from build123d import *

# Parameters (mm, degrees)
CROQUIS3_W                   = 38
CROQUIS3_H                   = 38
SALIENTE_EXTRUIR9_DEPTH      = 1
SALIENTE_EXTRUIR10_START     = -11
SALIENTE_EXTRUIR10_OUTLINE_W = 38
SALIENTE_EXTRUIR10_OUTLINE_H = 38
SALIENTE_EXTRUIR10_DEPTH     = 10
REDONDEO3_R                  = 1
CROQUIS13_W                  = 38
CROQUIS13_H                  = 38
SALIENTE_EXTRUIR15_DEPTH     = 3
CROQUIS15_R                  = 1.5
CORTAR_EXTRUIR5_DEPTH        = 5


# Read off the part's stored shape, not the designer's step: Saliente-Extruir10
with BuildPart() as part:
    # Croquis3 → Saliente-Extruir9 (new body)
    with BuildSketch(Plane.XY.offset(5)):
        Polygon((19, -5.370057685), (26.870057685, 2.5), (26.870057685, 40.5), (19, 48.370057685), (-19, 48.370057685), (-26.870057685, 40.5), (-26.870057685, 2.5), (-19, -5.370057685), align=None)
        with Locations((0, 21.5)):
            Rectangle(CROQUIS3_W, CROQUIS3_H, mode=Mode.SUBTRACT)
    extrude(amount=-SALIENTE_EXTRUIR9_DEPTH)

    # Saliente-Extruir10 outline → Saliente-Extruir10 (add)
    with BuildSketch(Plane(origin=(0, 0, 4), x_dir=(-1, 0, 0), z_dir=(0, 0, -1)).offset(SALIENTE_EXTRUIR10_START)):
        Polygon((-26.870057685, 2.5), (-19, -5.370057685), (19, -5.370057685), (26.870057685, 2.5), (26.870057685, 40.5), (19, 48.370057685), (-19, 48.370057685), (-26.870057685, 40.5), align=None)
        with Locations((0, 21.5)):
            Rectangle(SALIENTE_EXTRUIR10_OUTLINE_W, SALIENTE_EXTRUIR10_OUTLINE_H, mode=Mode.SUBTRACT)
    extrude(amount=SALIENTE_EXTRUIR10_DEPTH)

    # Redondeo3
    redondeo3_edges = [part.edges().sort_by_distance(p)[0] for p in [
        (-19, 48.370057685, 10),
        (19, 48.370057685, 10),
    ]]
    fillet(redondeo3_edges, radius=REDONDEO3_R)

    # Croquis13 → Saliente-Extruir15 (add)
    with BuildSketch(Plane.XY.offset(15)):
        with BuildLine():
            Line((-22.5, 44.870057685), (-22.5, -1))
            Line((-22.5, -1), (22.5, -1))
            Line((22.5, -1), (22.5, 44.870057685))
            Line((22.5, 44.870057685), (19.292893219, 48.077164466))
            ThreePointArc((19.292893219, 48.077164466), (18.96846987, 48.293937218), (18.585786438, 48.370057685))
            Line((18.585786438, 48.370057685), (-18.585786438, 48.370057685))
            ThreePointArc((-18.585786438, 48.370057685), (-18.96846987, 48.293937218), (-19.292893219, 48.077164466))
            Line((-19.292893219, 48.077164466), (-22.5, 44.870057685))
        make_face()
        with Locations((0, 21.5)):
            Rectangle(CROQUIS13_W, CROQUIS13_H, mode=Mode.SUBTRACT)
    extrude(amount=SALIENTE_EXTRUIR15_DEPTH)

    # Croquis15 → Cortar-Extruir5 (cut)
    with BuildSketch(Plane(origin=(0, 48.370057685, 0), x_dir=(1, 0, 0), z_dir=(0, 1, 0))):
        with Locations(Location((0, -12.5, 0), (0, 0, 270))):
            Circle(CROQUIS15_R)
        with Locations(Location((-10, -12.5, 0), (0, 0, 270))):
            Circle(CROQUIS15_R)
        with Locations(Location((10, -12.5, 0), (0, 0, 90))):
            Circle(CROQUIS15_R)
    extrude(amount=-CORTAR_EXTRUIR5_DEPTH, mode=Mode.SUBTRACT)


solid = part.part
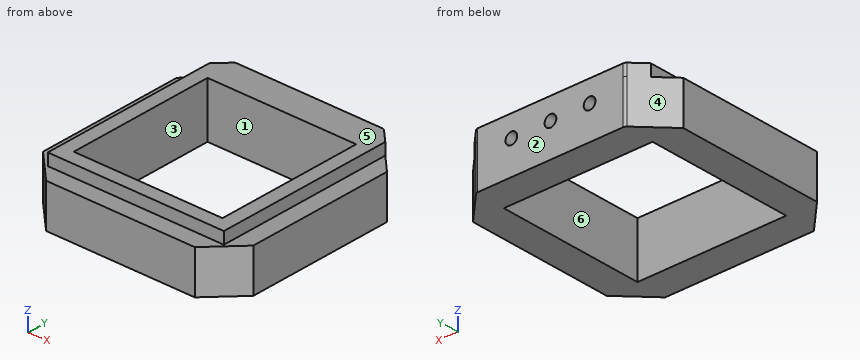
Part model, mm, in its own coordinate system. Face numbers are marked on the shaded views. A direction names the side the tool comes from. Coordinates: 2 decimals unless noted, no trailing zeros. Loops run counter-clockwise (first coordinate to the right, second up) from the corner with the lowest first, then second, coordinate; pieces in that order, holes last. Notation, with made-up numbers: (-19.5, 44) -> (24.5, 44) arc R24 cw to (24.5, 79) -> close; hole circle Ø1 at (-28.75, 41). An arc over 180 degrees is marked (long way). Use a Markdown table: item, result. Add a question column.
Item 1: Band-saw the part on D-D on y = 44. Write the cut outline in (x, z).
Item 2: Which spindle directions (+Z, -Z, +X, -X, +Y, -Y) get a long thin tool onto all of the face, cutting with end or side? Do the marked faces 1 and 2. Say none if no direction does.
Item 3: Pull direction X, two halves, no side cores. Call the marked faces 3, 4, 5 and 6: +X half, -X half, draft (parallel to the pull), parting line (faces both ways), or undercut.
Item 4: Probe probe 1 along X at (y, z) = (12, 6.5); probe 2 along X at (y, z) = (3, 16.5); probe 3 along X at (y, z) = (45.2, 12.5). List the from-to ranges inside material, lowest first.
Item 5: Band-saw the part on A-A on y = 4. Write the cut outline in (x, z), plus the area to 3 significant figures.
Item 6: Band-saw the part on B-B on x = 10. Write the cut outline in (y, z).
Item 7: Band-saw the part on C-C on z = 5.75. Write the cut outline in (x, y), plus the area to 3 significant figures.
Item 8: Flat gauge pins, fed straight in: P1, Ø2.5, axis at x = 10, z = 12.5, coming from the +Y side; P2, Ø25, axis at x = 0.5, y = 22.5, coming from the +Z side; P3, Ø3.5, axis at x = 7, z = 17, coming from the -Y side; P4, Ø1.5, axis at y = 20.5, z = 16, coming from the -X side. Where does each tip first touch, or does it go through?
Geometry says:
| question | item | result |
|---|---|---|
| 1 | outline | (-23.37, 4) -> (23.37, 4) -> (23.37, 15) -> (22.5, 15) -> (22.5, 18) -> (-22.5, 18) -> (-22.5, 15) -> (-23.37, 15) -> close; hole circle Ø3 at (-10, 12.5); hole circle Ø3 at (0, 12.5); hole circle Ø3 at (10, 12.5) |
| 2 | face 1 | +Z, -Z |
| 2 | face 2 | +Z, -Z, +X, -X, +Y |
| 3 | face 3 | undercut |
| 3 | face 4 | -X half |
| 3 | face 5 | draft |
| 3 | face 6 | undercut |
| 4 | probe 1 | -26.87 to -19, 19 to 26.87 |
| 4 | probe 2 | -22.5 to -19, 19 to 22.5 |
| 4 | probe 3 | -22.17 to -11.5, -8.5 to -1.5, 1.5 to 8.5, 11.5 to 22.17 |
| 5 | outline | (-26.87, 4) -> (-19, 4) -> (-19, 18) -> (-22.5, 18) -> (-22.5, 15) -> (-26.87, 15) -> close; (19, 4) -> (26.87, 4) -> (26.87, 15) -> (22.5, 15) -> (22.5, 18) -> (19, 18) -> close |
| 5 | area | 194 mm² |
| 6 | outline | (-5.37, 4) -> (2.5, 4) -> (2.5, 18) -> (-1, 18) -> (-1, 15) -> (-5.37, 15) -> close; (40.5, 4) -> (48.37, 4) -> (48.37, 11) -> (43.37, 11) -> (43.37, 14) -> (48.37, 14) -> (48.37, 18) -> (40.5, 18) -> close |
| 7 | outline | (-26.87, 2.5) -> (-19, -5.37) -> (19, -5.37) -> (26.87, 2.5) -> (26.87, 40.5) -> (19.29, 48.08) arc R1 ccw to (18.59, 48.37) -> (-18.59, 48.37) arc R1 ccw to (-19.29, 48.08) -> (-26.87, 40.5) -> close; hole (-19, 2.5) -> (19, 2.5) -> (19, 40.5) -> (-19, 40.5) -> close |
| 7 | area | 1,320 mm² |
| 8 | P1 | y = 43.37 |
| 8 | P2 | through |
| 8 | P3 | y = -1 |
| 8 | P4 | x = -22.5 |
